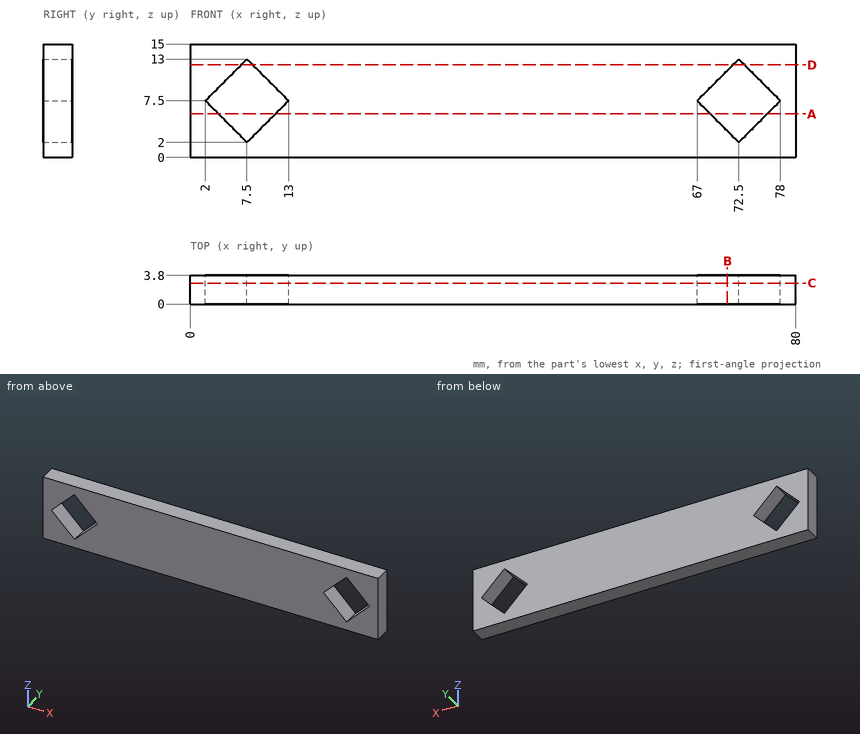
Study the drawing (mm; zero at the part's minimum x, y, z) and answer. Round coordinates to 2 decimals unless told otherwise and drop trailing zeros. Loops run counter-clockwise (first coordinate to the right, second up) from the corner with the lowest first, then second, coordinate; pieces in that order, holes last.
Q1. Section D-D, the plane z = 12.25 is taken. Determine the outline of the cut face in (x, y), then the cut area to 3 significant figures.
Q2. Section B-B, the plane x = 71 is taken. Determine the outline of the cut face in (y, z).
Q3. Section C-C, the plane y = 2.8 is taken. Determine the outline of the cut face in (x, z).
Q4. Section A-A, the plane z = 5.75 is taken. Determine the outline of the cut face in (x, y).
Q5. Find the intervals of material crossed by line 1 (X direction, y = 1, z = 5); line 2 (X direction, y = 1.45, z = 5.75); line 3 (Z direction, x = 6.5, y = 3.6), in increasing order.
Completed:
1. outline: (0, 0) - (6.75, 0) - (6.75, 3.8) - (0, 3.8) - close; (8.25, 0) - (71.75, 0) - (71.75, 3.8) - (8.25, 3.8) - close; (73.25, 0) - (80, 0) - (80, 3.8) - (73.25, 3.8) - close
1. area: 293 mm2
2. outline: (0, 0) - (3.8, 0) - (3.8, 3.5) - (0, 3.5) - close; (0, 11.5) - (3.8, 11.5) - (3.8, 15) - (0, 15) - close
3. outline: (0, 0) - (80, 0) - (80, 15) - (0, 15) - close; hole (2, 7.5) - (7.5, 2) - (13, 7.5) - (7.5, 13) - close; hole (67, 7.5) - (72.5, 2) - (78, 7.5) - (72.5, 13) - close
4. outline: (0, 0) - (3.75, 0) - (3.75, 3.8) - (0, 3.8) - close; (11.25, 0) - (68.75, 0) - (68.75, 3.8) - (11.25, 3.8) - close; (76.25, 0) - (80, 0) - (80, 3.8) - (76.25, 3.8) - close
5. line 1: x = 0 to 4.5, 10.5 to 69.5, 75.5 to 80
5. line 2: x = 0 to 3.75, 11.25 to 68.75, 76.25 to 80
5. line 3: z = 0 to 3, 12 to 15
